from build123d import *

# Parameters (mm, degrees)
SKETCH1_W           = 102.7938
SKETCH1_H           = 76.2
BOSS_EXTRUDE1_DEPTH = 38.1
SKETCH2_W           = 96.4438
SKETCH2_H           = 69.85
CUT_EXTRUDE1_DEPTH  = 25.4
SKETCH3_W           = 3.048
SKETCH3_H           = 3.302
BOSS_EXTRUDE2_DEPTH = 25.4
FILLET1_R           = 38.1
SKETCH8_W           = 10.668
SKETCH8_H           = 10.668
CUT_EXTRUDE3_DEPTH  = 19.05
SKETCH7_W           = 102.7938
SKETCH7_H           = 76.2
CUT_EXTRUDE4_DEPTH  = 7.62
FILLET2_R           = 38.1
SKETCH9_W           = 3.048
SKETCH9_H           = 3.302
BOSS_EXTRUDE3_DEPTH = 12.7
SKETCH10_W          = 2
SKETCH10_H          = 76.2
BOSS_EXTRUDE4_DEPTH = 1
FILLET3_R           = 0.9


with BuildPart() as part:
    # Sketch1 → Boss-Extrude1 (new body)
    with BuildSketch(Plane(origin=(0, 0, 0), x_dir=(1, 0, 0), z_dir=(0, 1, 0))):
        with Locations((51.3969, 38.1)):
            Rectangle(SKETCH1_W, SKETCH1_H)
    extrude(amount=BOSS_EXTRUDE1_DEPTH)

    # Sketch2 → Cut-Extrude1 (cut)
    with BuildSketch(Plane(origin=(0, 38.1, 0), x_dir=(1, 0, 0), z_dir=(0, 1, 0))):
        with Locations((51.3969, 38.1)):
            Rectangle(SKETCH2_W, SKETCH2_H)
    extrude(amount=-CUT_EXTRUDE1_DEPTH, mode=Mode.SUBTRACT)

    # Sketch3 → Boss-Extrude2 (add, symmetric)
    with BuildSketch(Plane.XZ):
        with Locations((0.9779, -24.524)):
            Rectangle(SKETCH3_W, SKETCH3_H)
        with Locations((101.8159, -24.524)):
            Rectangle(SKETCH3_W, SKETCH3_H)
    extrude(amount=BOSS_EXTRUDE2_DEPTH, both=True)

    # Fillet1
    # the kernel refuses this fillet: 38.1 mm, written as the material it adds along each edge
    with BuildSketch(Plane(origin=(3.175, 12.7, -3.175), x_dir=(0, 1, 0), z_dir=(1, 0, 0)), Plane(origin=(99.6188, 12.7, -73.025), x_dir=(0, 1, 0), z_dir=(-1, 0, 0))) as fillet1_piece_1:
        with BuildLine():
            CenterArc((38.1, -35.921024484), FILLET1_R, 109.471220634, 70.528779366)
            Line((0, -35.921024484), (-0.762, -35.921024484))
            Line((-0.762, -35.921024484), (-0.762, 0))
            Line((-0.762, 0), (0, 0.762))
            ThreePointArc((0, 0.762), (12.7, 0.762), (25.146, 0.71842049))
            Line((25.146, 0.71842049), (25.4, 0))
        make_face()
    extrude(amount=96.4438)

    # Sketch8 → Cut-Extrude3 (cut)
    with BuildSketch(Plane(origin=(0, 38.1, 0), x_dir=(1, 0, 0), z_dir=(0, 1, 0))):
        with Locations((51.3969, 67.691)):
            Rectangle(SKETCH8_W, SKETCH8_H)
    extrude(amount=-CUT_EXTRUDE3_DEPTH, mode=Mode.SUBTRACT)

    # Sketch7 → Cut-Extrude4 (cut)
    with BuildSketch(Plane(origin=(0, 38.1, 0), x_dir=(1, 0, 0), z_dir=(0, 1, 0))):
        with Locations((51.3969, 38.1)):
            Rectangle(SKETCH7_W, SKETCH7_H)
    extrude(amount=-CUT_EXTRUDE4_DEPTH, mode=Mode.SUBTRACT)

    # Fillet2
    # the kernel refuses this fillet: 38.1 mm, written as the material it adds along each edge
    with BuildSketch(Plane(origin=(0, 25.4, -22.873), x_dir=(0, 0, 1), z_dir=(0, -1, 0)), Plane(origin=(0, 0, -26.175), x_dir=(0, 0, -1), z_dir=(0, 1, 0))) as fillet2_piece_1:
        with BuildLine():
            CenterArc((6.42764302, 38.1), FILLET2_R, 260.287493111, 9.712506889)
            Line((0, 0.5461), (0, 0))
            Line((0, 0), (6.42764302, 0))
        make_face()
    extrude(amount=25.4)
    with BuildSketch(Plane(origin=(102.7938, 0, -26.175), x_dir=(0, 0, -1), z_dir=(0, 1, 0)), Plane(origin=(102.7938, 25.4, -22.873), x_dir=(0, 0, 1), z_dir=(0, -1, 0))) as fillet2_piece_2:
        with BuildLine():
            CenterArc((6.42764302, -38.1), FILLET2_R, 90, 9.712506889)
            Line((0, -0.5461), (0, 0))
            Line((0, 0), (6.42764302, 0))
        make_face()
    extrude(amount=25.4)

    # Sketch9 → Boss-Extrude3 (add)
    with BuildSketch(Plane.XZ.offset(25.4)):
        with Locations((0.9779, -24.524)):
            Rectangle(SKETCH9_W, SKETCH9_H)
        with Locations((101.8159, -24.524)):
            Rectangle(SKETCH9_W, SKETCH9_H)
    extrude(amount=BOSS_EXTRUDE3_DEPTH)

    # Sketch10 → Boss-Extrude4 (add)
    with BuildSketch(Plane.XZ):
        with Locations((51.3969, -38.1)):
            Rectangle(SKETCH10_W, SKETCH10_H)
    extrude(amount=BOSS_EXTRUDE4_DEPTH)

    # Fillet3
    fillet3_edges = [part.edges().sort_by_distance(p)[0] for p in [
        (50.3969, 0, -38.1),
        (52.3969, 0, -38.1),
    ]]
    fillet(fillet3_edges, radius=FILLET3_R)


solid = part.part
The listing builds one solid part. Answer for the finished solid, in the listing's coordinates (mm). A direction names the side the tool comes from. Coordinates: 2 decimals unless noted, no trailing zeros. Write each loop counter-clockwise with the first axis right and the second up, starting at its lowest first coordinate (ties: lowest second). Pieces come first, ordered by that corner, then holes. Notation, with made-up numbers: M 76,69 L 113,69 A9 cw 113,77 Z; hole C 62.5,68.25 d4. An arc over 180 degrees is marked long. Put each result on its own line as item: value. Start each with the question number.
1. Flat-ended cylindrical pins translate along their axes: P1, Ø10, axis at x = 77.5, z = -35.5, coming from the +Y side; P2, Ø1, axis at x = 71.5, z = -42, coming from the -Y side; P3, Ø2, axis at y = 11.5, z = -45.5, coming from the +X side. Find the tip coordinate at first contact, or state that the pin passes through.
2. A cutting plane is placed at D-D on x = 47.5. Write down the section's boundary in (y, z) (3 decimals).
3. A cutting plane is placed at A-A on y = -11. Write down the section's boundary in (x, z) (3 decimals), then the cut area to 3 significant figures.
4. Consider line 1 (X direction, y = 23.5, z = -52.5) (3 decimals); line 2 (Y direction, x = 15, z = -70); line 3 (Z direction, x = 55, y = 16). Determine where each line is inside the solid, lowest interval first. Write a range as from..to.
5. For a pull along Z with two mould halves and no side action, classify faces 3 (the flat face through (99.619, 24, -38)), 4 (the flat face through (102, -19, -22.873)), 5 (the flat face through (1, -19, -26.175)), 6 (the flat face through (51, 21, -62.357)) as pulls with the +Z half, pulls with the -Z half, needs draft (parallel to the pull), parting line crosses it, or undercut.
6. A cutting plane is placed at B-B on x = 58. Write down the section's boundary in (y, z).
7. Which of the six approach directions +Z, -Z, +X, -X, +Y, -Y give full straight-line access (tool end or side, diameter ignored) to faces 1 (the flat face through (3.175, 24, -38)), 2 (the cylindrical face through (102.927, 12.522, -29.422))?
8. A cutting plane is placed at C-C on z = -61. Write down the section's boundary in (x, y) (3 decimals), then the cut area to 3 significant figures.
Resolved:
1. P1: stops at y = 13.68
1. P2: stops at y = 0
1. P3: stops at x = 102.79
2. outline: M 0,-76.2 L 30.48,-76.2 L 30.48,-73.025 L 19.05,-73.025 L 19.05,-62.357 L 22.271,-62.357 A38.1 cw 12.713,-38.1 A38.1 cw 30.48,-6.867 L 30.48,0 L 0,0 Z
3. outline: M -0.546,-26.175 L 2.502,-26.175 L 2.502,-22.873 L -0.546,-22.873 Z; M 100.292,-26.175 L 103.34,-26.175 L 103.34,-22.873 L 100.292,-22.873 Z
3. area: 20.1 mm2
4. line 1: x = 0..3.175, 99.619..102.794
4. line 2: y = 0..30.48
4. line 3: z = -76.2..-52.61, -23.59..0
5. face 3: undercut
5. face 4: pulls with the +Z half
5. face 5: pulls with the -Z half
5. face 6: undercut
6. outline: M 0,-76.2 L 30.48,-76.2 L 30.48,-69.33 A38.1 cw 12.71,-38.1 A38.1 cw 30.48,-6.87 L 30.48,0 L 0,0 Z
7. face 1: +Y
7. face 2: -Z, +X, +Y, -Y
8. outline: M 0,0 L 49.497,0 A0.9 cw 50.397,-0.9 L 50.397,-1 L 52.397,-1 L 52.397,-0.9 A0.9 cw 53.297,0 L 102.794,0 L 102.794,30.48 L 99.619,30.48 L 99.619,21.125 L 3.175,21.125 L 3.175,30.48 L 0,30.48 Z
8. area: 2,230 mm2
